Autodesk Inventor part; units mm, degrees
ref_plane "YZ Plane" through (0, 0, 0) normal (1, 0, 0) x (0, 1, 0)
ref_plane "XZ Plane" through (0, 0, 0) normal (0, 1, 0) x (-1, 0, 0)
ref_plane "XY Plane" through (0, 0, 0) normal (0, 0, 1) x (1, 0, 0)
sketch "Sketch1" plane through (0, 0, 0) normal (0, 1, 0) x (-1, 0, 0)
  line L0 (0, 0) -> (0, 25)
  line L1 (0, 0) -> (-25, 0)
  line L2 (0, 0) -> (0, -25)
  line L3 (0, 0) -> (25, 0)
  line L4 (25, 0) -> (25, -9)
  line L5 (0, -25) -> (9, -25)
  line L6 (9, -25) -> (9, -9)
  line L7 (9, -9) -> (25, -9)
  line L8 (0, -25) -> (-9, -25)
  line L9 (-9, -25) -> (-9, -9)
  line L10 (-9, -9) -> (-25, -9)
  line L11 (-25, -9) -> (-25, 0)
  line L12 (-25, 0) -> (-25, 9)
  line L13 (-25, 9) -> (-9, 9)
  line L14 (-9, 9) -> (-9, 25)
  line L15 (-9, 25) -> (0, 25)
  line L16 (9, 25) -> (0, 25)
  line L17 (9, 25) -> (9, 9)
  line L18 (9, 9) -> (25, 9)
  line L19 (25, 9) -> (25, 0)
  line L20 (21.8, -5.8) -> (5.8, -5.8)
  line L21 (5.8, -5.8) -> (5.8, -21.8)
  line L22 (5.8, -21.8) -> (-5.8, -21.8)
  line L23 (-5.8, -21.8) -> (-5.8, -5.8)
  line L24 (-5.8, -5.8) -> (-21.8, -5.8)
  line L25 (-21.8, -5.8) -> (-21.8, 5.8)
  line L26 (-21.8, 5.8) -> (-5.8, 5.8)
  line L27 (-5.8, 5.8) -> (-5.8, 21.8)
  line L28 (-5.8, 21.8) -> (5.8, 21.8)
  line L29 (5.8, 21.8) -> (5.8, 5.8)
  line L30 (5.8, 5.8) -> (21.8, 5.8)
  line L31 (21.8, 5.8) -> (21.8, -5.8)
  dimension "d0" = 25
  dimension "d1" = 25
  dimension "d2" = 25
  dimension "d3" = 25
  dimension "d4" = 9
  dimension "d5" = 9
  dimension "d6" = 9
  dimension "d7" = 9
  dimension "d8" = 9
  dimension "d9" = 9
  dimension "d10" = 9
  dimension "d11" = 9
  dimension "d34" = 3.2
  dimension "d35" = 3.2
  dimension "d36" = 3.2
  dimension "d37" = 3.2
  dimension "d38" = 3.2
  dimension "d39" = 3.2
  dimension "d40" = 3.2
  dimension "d41" = 3.2
  dimension "d42" = 3.2
  dimension "d43" = 3.2
  dimension "d44" = 3.2
  dimension "d45" = 3.2
extrude "Extrusion1" add sketch "Sketch1" along normal blind 4.8 contours L1 L25 L26 L27 L28 L0 | L2 L22 L23 L24 L25 L1 | L3 L31 L20 L21 L22 L2 | L0 L28 L29 L30 L31 L3
sketch "Sketch3" plane through (0, 4.8, 0) normal (0, 1, 0) x (1, 0, 0)
  circle A0 centre (0, 0) radius 4.1
  dimension "d18" = 8.2
extrude "Extrusion3" add sketch "Sketch3" along normal blind 8
sketch "Sketch6" plane through (0, 4.8, 0) normal (0, 1, 0) x (1, 0, 0)
  circle A0 centre (0, 0) radius 7.5
  dimension "d31" = 15
extrude "Extrusion6" add sketch "Sketch6" along normal blind 3
sketch "Sketch4" plane through (0, 12.8, 0) normal (0, 1, 0) x (1, 0, 0)
  line L0 (-0.0005, -0.0003) -> (-0.0005, -1.7003)
  line L1 (-0.0005, -1.7003) -> (2.6995, -1.7003)
  line L2 (2.6995, -1.7003) -> (2.6995, 1.6997)
  line L3 (2.6995, 1.6997) -> (-2.7005, 1.6997)
  line L4 (-2.7005, 1.6997) -> (-2.7005, -1.7003)
  line L5 (-2.7005, -1.7003) -> (-0.0005, -1.7003)
  point P0 (0, 0)
  dimension "d21" = 1.7
  dimension "d22" = 2.7
  dimension "d23" = 3.4
  dimension "d24" = 5.4
extrude "Extrusion4" cut sketch "Sketch4" against normal blind 8.2
sketch "Sketch5" plane through (0, 12.8, 0) normal (0, 1, 0) x (1, 0, 0)
  circle A0 centre (0, 0) radius 2.7
  dimension "d27" = 5.4
extrude "Extrusion5" cut sketch "Sketch5" against normal blind 2.2
fillet "Fillet1" radius 0.635 4 edges at (-2.7005, 8.7, -1.6997) (-2.7005, 8.7, 1.7003) (2.6995, 8.7, -1.6997) (2.6995, 8.7, 1.7003)
equation "\"d5\" = d4"
equation "\"d6\" = d4"
equation "\"d7\" = d4"
equation "\"d35\" = d34"
equation "\"d36\" = d34"
equation "\"d37\" = d34"
equation "\"d38\" = d34"
equation "\"d39\" = d34"
equation "\"d40\" = d34"
equation "\"d41\" = d34"
equation "\"d42\" = d34"
equation "\"d44\" = d34"
equation "\"d21\" = 0.5 * d23"
properties part number "Motor_Key_Cross"
Build history of the part. All positions in model axes, mm. A direction names the side the tool comes from. Coordinates: 2 decimals unless noted, no trailing zeros. Write each loop counter-clockwise with the first axis right and the second up, starting at its lowest first coordinate (ties: lowest second). Pieces come first, ordered by that corner, then holes.
(1) Pin check, flat tips, straight feed: pin 1 Ø1.1 at (y, z) = (7, 0.5) entering from -X; pin 2 Ø3.5 at (x, y) = (-0.5, 6.5) entering from +Z; pin 3 Ø5.5 at (x, y) = (17, 1.5) entering from +Z; pin 4 Ø5 at (x, z) = (9, -14) entering from -Y. Stop position of each tip, or through.
(2) Cut at B-B on x = 0. List the corners of the cut face in (y, z).
(3) Cut at C-C on z = 13. List the corners of the cut face in (x, y), and give its area (3 significant figures).
(4) 3-axis set-ups, long thin cutter, end or side, ignore diameter. For faces 1 (the flat face through (-5.8, 2, 14)), 2 (the flat face through (-2.7, 9, 0)), 3 (the flat face through (0, 2, 21.8)), 4 (the flat face through (-14, 2, -5.8)), 5 (the flat face through (14, 2, 5.8)): which of +Z, -Z, +X, -X, +Y, -Y reach the whole face in a straight line?
(5) Cut at A-A on y = 4. List the corners of the cut face in (x, z).
(6) Mould opens along Z. For faces 6 (the cylindrical face through (-7.493, 6.279, 0.33)), 7 (the flat face through (0, 8, -1.7)), 8 (the flat face through (-21.8, 2, 0)) say: pulls with the +Z half, pulls with the -Z half, needs draft (parallel to the pull), parting line crosses it, or undercut.
(7) Drill centre lines: line 1 (Y direction, x = 9, z = -4); line 2 (X direction, y = 1, z = 14). Where is each one in solid material? Low to high.
Working result:
1. pin 1: stops at x = -7.5
1. pin 2: stops at z = 21.8
1. pin 3: stops at z = 5.8
1. pin 4: passes through
2. outline: (0, -21.8) - (4.8, -21.8) - (4.8, -7.5) - (7.8, -7.5) - (7.8, -4.1) - (12.8, -4.1) - (12.8, -2.7) - (10.6, -2.7) - (10.6, -1.7) - (4.6, -1.7) - (4.6, 1.7) - (10.6, 1.7) - (10.6, 2.7) - (12.8, 2.7) - (12.8, 4.1) - (7.8, 4.1) - (7.8, 7.5) - (4.8, 7.5) - (4.8, 21.8) - (0, 21.8) - close
3. outline: (-5.8, 0) - (5.8, 0) - (5.8, 4.8) - (-5.8, 4.8) - close
3. area: 55.7 mm2
4. face 1: +Z, -X, +Y, -Y
4. face 2: +Y
4. face 3: +Z, +X, -X, +Y, -Y
4. face 4: -Z, -X, +Y, -Y
4. face 5: +Z, +X, +Y, -Y
5. outline: (-21.8, -5.8) - (-5.8, -5.8) - (-5.8, -21.8) - (5.8, -21.8) - (5.8, -5.8) - (21.8, -5.8) - (21.8, 5.8) - (5.8, 5.8) - (5.8, 21.8) - (-5.8, 21.8) - (-5.8, 5.8) - (-21.8, 5.8) - close
6. face 6: parting line crosses it
6. face 7: undercut
6. face 8: needs draft
7. line 1: y = 0 to 4.8
7. line 2: x = -5.8 to 5.8
